```python
from build123d import *

# Parameters (mm, degrees)
F1_DEPTH = 12.7
F0_W     = 17.78
F0_H     = 2.54
F0_W_2   = 28.5250723219
F0_H_2   = 12.6543707534
F0_H_3   = 4.4012725921
F2_DEPTH = 25.4
F3_R     = 5.08


with BuildPart() as f1:
    # F0 (on Front) → F1 (new body)
    with BuildSketch(Plane.XZ):
        Polygon((8.89, 33.02), (-8.89, 33.02), (-8.89, -33.02), (8.89, -33.02), (8.89, -4.1522149311), (8.89, 8.5021558223), align=None)
    extrude(amount=F1_DEPTH)

    # F0 (on Front) → F2 (join)
    with BuildSketch(Plane.XZ):
        Polygon((8.89, 33.02), (-8.89, 33.02), (-8.89, -33.02), (8.89, -33.02), (8.89, -4.1522149311), (8.89, 8.5021558223), align=None)
        with Locations((0, -34.29)):
            Rectangle(F0_W, F0_H)
        with Locations((23.1525361609, 2.1749704456)):
            Rectangle(F0_W_2, F0_H_2)
        Polygon((37.4150723219, 30.48), (37.4150723219, 8.5021558223), (37.4150723219, -4.1522149311), (37.4150723219, -31.1587274079), (55.1950723219, -31.1587274079), (55.1950723219, 30.48), align=None)
        with Locations((46.3050723219, -33.359363704)):
            Rectangle(F0_W, F0_H_3)
    extrude(amount=F2_DEPTH)

    # F3
    f3_edges = [f1.edges().sort_by_distance(p)[0] for p in [
        (55.195072, -25.4, -2.54),
        (55.195072, 0, -2.54),
        (37.415072, -25.4, 19.491078),
        (8.89, -25.4, 20.761078),
        (8.89, -25.4, -19.856107),
        (-8.89, -25.4, -1.27),
        (23.152536, -25.4, 8.502156),
        (23.152536, -25.4, -4.152215),
        (37.415072, 0, -19.856107),
        (37.415072, 0, 19.491078),
        (23.152536, 0, -4.152215),
        (8.89, 0, 20.761078),
        (8.89, 0, -19.856107),
        (-8.89, 0, -1.27),
    ]]
    fillet(f3_edges, radius=F3_R)


solid = f1.part
```
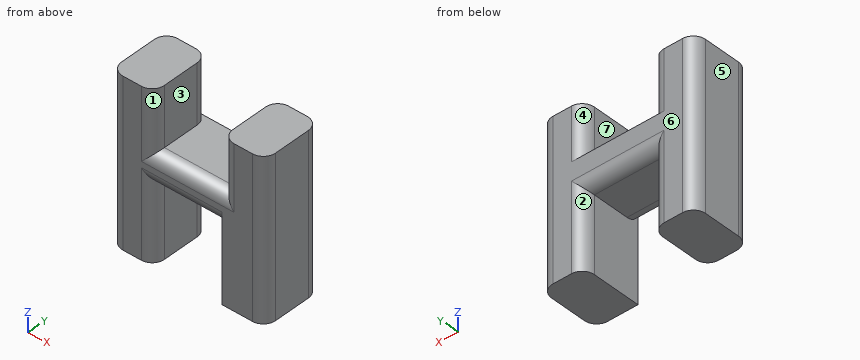
Here's how the part is built. I have some questions about the finished solid (model axes, mm). Face numbers are marked on the shaded views. A direction names the side the tool comes from. Give positions to 0.01 mm unless a question says otherwise; leave off trailing zeros. Write each loop counter-clockwise with the first axis right and the second up, starting at its lowest first coordinate (ties: lowest second). Pieces come first, ordered by that corner, then holes. Notation, with made-up numbers: M -3,-18 L 40,-18 A30 cw 40,9 Z; hole C -18.5,-5.5 d2. An arc over 180 degrees is marked long. Put each result on its own line as item: value. Start each with the question number.
Item 1: If we section it at C-C, the plane y = -8.75: Write out the boundary of the cut face in (x, z), then the cut area to 3 significant figures.
Item 2: Will these pins go through, and if not, where does the flat tip stop? pin 1 (12 mm diameter, centred on x = 25, y = -16, fed in from -Z); pin 2 (8 mm diameter, centred on x = 36, y = -19, fed in from +Z); pin 3 (2 mm diameter, centred on x = 33.5, y = -3.5, fed in from -Z).
Item 3: If we section it at B-B, the plane z = 22: Write out the boundary of the cut face in (x, y), then the cut area to 3 significant figures.
Item 4: On a 3-axis mill with a long thin cutter (end or side, diameter ignored), from which of +Z, -Z, +X, -X, +Y, -Y can I reach the whole of each face in a straight line? I mean the marked faces 1, 2, 3 and 4. Say none if no direction works.
Item 5: If we section it at A-A, the plane z = -6: Write out the boundary of the cut face in (x, y), then the cut area to 3 significant figures.
Item 6: Thinking about a two-plate mould opening in X: for the marked faces 5, 6 and 7, which applies, +X half, -X half, draft (parallel to the pull), parting line (faces both ways), or undercut?
Item 7: I need wall thicknesses on L1, parallel to X at y = -15.75, z = 11; L2, parallel to Z at x = 10, y = -15.5; L3, parallel to X at y = -3, z = 16.5. Which ranges of each line are inside material? Lowest first, please. Write a range as from..to.
Item 8: If we section it at D-D, the plane x = 27.5: Write out the boundary of the cut face in (y, z).
Values:
1. outline: M -8.89,-35.56 L 8.89,-35.56 L 8.89,-4.15 L 37.42,-4.15 L 37.42,-35.56 L 55.2,-35.56 L 55.2,30.48 L 37.42,30.48 L 37.42,8.5 L 8.89,8.5 L 8.89,33.02 L -8.89,33.02 Z
1. area: 2,750 mm²
2. pin 1: z = -4.15
2. pin 2: z = 30.48
2. pin 3: z = -4.12
3. outline: M -8.89,-20.32 A5.08 ccw -3.81,-25.4 L 3.81,-25.4 A5.08 ccw 8.89,-20.32 L 8.89,-5.08 A5.08 ccw 3.81,0 L -3.81,0 A5.08 ccw -8.89,-5.08 Z; M 37.42,-20.32 A5.08 ccw 42.5,-25.4 L 50.12,-25.4 A5.08 ccw 55.2,-20.32 L 55.2,-5.08 A5.08 ccw 50.12,0 L 42.5,0 A5.08 ccw 37.42,-5.08 Z
3. area: 859 mm²
4. face 1: +Z, -Y
4. face 2: -Z, +Y
4. face 3: +Z, +Y, -Y
4. face 4: +Z, +Y
5. outline: M -8.89,-20.32 A5.08 ccw -3.81,-25.4 L 3.81,-25.4 A5.08 ccw 8.89,-20.32 L 8.89,-5.08 A5.08 ccw 3.81,0 L -3.81,0 A5.08 ccw -8.89,-5.08 Z; M 37.42,-25.4 L 50.12,-25.4 A5.08 ccw 55.2,-20.32 L 55.2,-5.08 A5.08 ccw 50.12,0 L 42.5,0 A5.08 ccw 37.42,-5.08 Z
5. area: 864 mm²
6. face 5: -X half
6. face 6: draft
6. face 7: undercut
7. L1: -8.89..8.89, 37.42..55.2
7. L2: -4.15..8.5
7. L3: -8.44..8.44, 37.86..54.75
8. outline: M -25.4,0.93 A5.08 ccw -20.32,-4.15 L -5.08,-4.15 A5.08 ccw 0,0.93 L 0,8.5 L -20.32,8.5 A5.08 ccw -25.4,3.42 Z
